Design review of the part built by this model. Coordinates are the model's own, in mm. Face numbers are marked on the shaded views. A direction names the side the tool comes from. Give positions to 0.01 mm unless a question says otherwise; leave off trailing zeros. Write each loop counter-clockwise with the first axis right and the second up, starting at its lowest first coordinate (ties: lowest second). Pieces come first, ordered by that corner, then holes. Notation, with made-up numbers: M -24.75,53.25 L -12.75,53.25 A7 cw -12.75,58.25 Z; hole C 73,78 d1. An arc over 180 degrees is marked long. One line per item, written item: value. Start each with the question number.
```python
from build123d import *

# Parameters (mm, degrees)
SKETCH1_W            = 300
SKETCH1_H            = 20
BOSS_EXTRUDE1_DEPTH  = 8
SKETCH2_W            = 34
SKETCH2_H            = 8
BOSS_EXTRUDE2_DEPTH  = 9
SKETCH3_W            = 34
SKETCH3_H            = 8
BOSS_EXTRUDE3_DEPTH  = 9
SKETCH4_R            = 1.45
CUT_EXTRUDE1_DEPTH   = 302.504560496
SKETCH5_W            = 25
SKETCH5_H            = 8
BOSS_EXTRUDE4_DEPTH  = 17
SKETCH6_W            = 25
SKETCH6_H            = 8
BOSS_EXTRUDE5_DEPTH  = 17
SKETCH7_W            = 10
SKETCH7_H            = 38
CUT_EXTRUDE2_DEPTH   = 303.37890138
SKETCH8_W            = 7
SKETCH8_H            = 16
CUT_EXTRUDE3_DEPTH   = 4
CUT_EXTRUDE4_DEPTH   = 7
BOSS_EXTRUDE6_DEPTH  = 10
SKETCH12_W           = 8
SKETCH12_H           = 8
BOSS_EXTRUDE7_DEPTH  = 17
SKETCH13_R           = 1.7
CUT_EXTRUDE6_DEPTH   = 305.926220585
SKETCH14_W           = 20
SKETCH14_H           = 12
BOSS_EXTRUDE8_DEPTH  = 10
SKETCH15_R           = 1.6
CUT_EXTRUDE7_DEPTH   = 20
SKETCH16_W           = 20
SKETCH16_H           = 12
BOSS_EXTRUDE9_DEPTH  = 10
SKETCH17_R           = 1.6
CUT_EXTRUDE8_DEPTH   = 20
SKETCH18_W           = 20
SKETCH18_H           = 12
BOSS_EXTRUDE10_DEPTH = 10
CUT_EXTRUDE9_START   = -20
SKETCH19_R           = 1.6
CUT_EXTRUDE9_DEPTH   = 20
SKETCH20_W           = 20
SKETCH20_H           = 12
BOSS_EXTRUDE11_DEPTH = 10
CUT_EXTRUDE10_START  = -20
SKETCH21_R           = 1.6
CUT_EXTRUDE10_DEPTH  = 20
SKETCH22_W           = 207
SKETCH22_H           = 50
BOSS_EXTRUDE12_DEPTH = 8
SKETCH23_W           = 191
SKETCH23_H           = 44
CUT_EXTRUDE11_DEPTH  = 4
SKETCH24_W           = 10
SKETCH24_H           = 44
BOSS_EXTRUDE14_DEPTH = 19.4
SKETCH25_R           = 1.45
CUT_EXTRUDE12_DEPTH  = 15
FILLET1_R            = 5
FILLET2_R            = 5
FILLET3_R            = 8
FILLET4_R            = 15
FILLET5_R            = 25
FILLET6_R            = 3
SKETCH27_W           = 1.8
SKETCH27_H           = 5
CUT_EXTRUDE13_DEPTH  = 19.4


with BuildPart() as part:
    # Sketch1 → Boss-Extrude1 (new body)
    with BuildSketch(Plane(origin=(0, 0, 0), x_dir=(1, 0, 0), z_dir=(0, 1, 0))):
        with Locations((150, -10)):
            Rectangle(SKETCH1_W, SKETCH1_H)
    extrude(amount=BOSS_EXTRUDE1_DEPTH)

    # Sketch2 → Boss-Extrude2 (add)
    with BuildSketch(Plane.XY.offset(20)):
        with Locations((17, 4)):
            Rectangle(SKETCH2_W, SKETCH2_H)
        with Locations((283, 4)):
            Rectangle(SKETCH2_W, SKETCH2_H)
    extrude(amount=BOSS_EXTRUDE2_DEPTH)

    # Sketch3 → Boss-Extrude3 (add)
    with BuildSketch(Plane(origin=(0, 0, 0), x_dir=(-1, 0, 0), z_dir=(0, 0, -1))):
        with Locations((-17, 4)):
            Rectangle(SKETCH3_W, SKETCH3_H)
        with Locations((-283, 4)):
            Rectangle(SKETCH3_W, SKETCH3_H)
    extrude(amount=BOSS_EXTRUDE3_DEPTH)

    # Sketch4 → Cut-Extrude1 (cut, through all)
    with BuildSketch(Plane(origin=(0, 8, 0), x_dir=(1, 0, 0), z_dir=(0, 1, 0))):
        with Locations(Location((4, 5, 0), (0, 0, 270))):
            Circle(SKETCH4_R)
        with Locations(Location((30, 5, 0), (0, 0, 270))):
            Circle(SKETCH4_R)
        with Locations(Location((30, -25, 0), (0, 0, 270))):
            Circle(SKETCH4_R)
        with Locations(Location((4, -25, 0), (0, 0, 270))):
            Circle(SKETCH4_R)
        with Locations(Location((296, -25, 0), (0, 0, 270))):
            Circle(SKETCH4_R)
        with Locations(Location((296, 5, 0), (0, 0, 270))):
            Circle(SKETCH4_R)
        with Locations(Location((270, -25, 0), (0, 0, 270))):
            Circle(SKETCH4_R)
        with Locations(Location((270, 5, 0), (0, 0, 270))):
            Circle(SKETCH4_R)
    extrude(amount=-CUT_EXTRUDE1_DEPTH, mode=Mode.SUBTRACT)

    # Sketch5 → Boss-Extrude4 (add)
    with BuildSketch(Plane.XY.offset(20)):
        with Locations((253.5, 4)):
            Rectangle(SKETCH5_W, SKETCH5_H)
    extrude(amount=BOSS_EXTRUDE4_DEPTH)

    # Sketch6 → Boss-Extrude5 (add)
    with BuildSketch(Plane(origin=(0, 0, 0), x_dir=(-1, 0, 0), z_dir=(0, 0, -1))):
        with Locations((-253.5, 4)):
            Rectangle(SKETCH6_W, SKETCH6_H)
    extrude(amount=BOSS_EXTRUDE5_DEPTH)

    # Sketch7 → Cut-Extrude2 (cut, through all)
    with BuildSketch(Plane(origin=(0, 8, 0), x_dir=(1, 0, 0), z_dir=(0, 1, 0))):
        with Locations((254, -10)):
            Rectangle(SKETCH7_W, SKETCH7_H)
    extrude(amount=-CUT_EXTRUDE2_DEPTH, mode=Mode.SUBTRACT)

    # Sketch8 → Cut-Extrude3 (cut)
    with BuildSketch(Plane(origin=(0, 8, 0), x_dir=(1, 0, 0), z_dir=(0, 1, 0))):
        with Locations((262.5, -10)):
            Rectangle(SKETCH8_W, SKETCH8_H)
    extrude(amount=-CUT_EXTRUDE3_DEPTH, mode=Mode.SUBTRACT)

    # Sketch9 → Cut-Extrude4 (cut)
    with BuildSketch(Plane.ZY.offset(-259)):
        Polygon((18, 4), (22, 8), (18, 8), align=None)
        Polygon((2, 4), (-2, 8), (2, 8), align=None)
    extrude(amount=-CUT_EXTRUDE4_DEPTH, mode=Mode.SUBTRACT)

    # Sketch10 → Boss-Extrude6 (add)
    with BuildSketch(Plane.ZY.offset(-259)):
        Polygon((-2, 0), (-9, 8), (-9, 0), align=None)
        Polygon((29, 8), (22, 0), (29, 0), align=None)
    extrude(amount=BOSS_EXTRUDE6_DEPTH)

    # Sketch12 → Boss-Extrude7 (add)
    with BuildSketch(Plane.XY.offset(37)):
        with Locations((245, 4)):
            Rectangle(SKETCH12_W, SKETCH12_H)
    extrude(amount=BOSS_EXTRUDE7_DEPTH)

    # Sketch13 → Cut-Extrude6 (cut, through all)
    with BuildSketch(Plane(origin=(0, 8, 0), x_dir=(1, 0, 0), z_dir=(0, 1, 0))):
        with Locations(Location((245, -50, 0), (0, 0, 270))):
            Circle(SKETCH13_R)
        with Locations(Location((245, -18, 0), (0, 0, 270))):
            Circle(SKETCH13_R)
    extrude(amount=-CUT_EXTRUDE6_DEPTH, mode=Mode.SUBTRACT)

    # Sketch14 → Boss-Extrude8 (add)
    with BuildSketch(Plane.XY.offset(29)):
        with Locations((285, 6)):
            Rectangle(SKETCH14_W, SKETCH14_H)
    extrude(amount=BOSS_EXTRUDE8_DEPTH)

    # Sketch15 → Cut-Extrude7 (cut)
    with BuildSketch(Plane(origin=(295, 0, 0), x_dir=(0, 0, -1), z_dir=(1, 0, 0))):
        with Locations((-35, 8)):
            Circle(SKETCH15_R)
    extrude(amount=-CUT_EXTRUDE7_DEPTH, mode=Mode.SUBTRACT)

    # Sketch16 → Boss-Extrude9 (add)
    with BuildSketch(Plane(origin=(0, 0, -9), x_dir=(-1, 0, 0), z_dir=(0, 0, -1))):
        with Locations((-285, 6)):
            Rectangle(SKETCH16_W, SKETCH16_H)
    extrude(amount=BOSS_EXTRUDE9_DEPTH)

    # Sketch17 → Cut-Extrude8 (cut)
    with BuildSketch(Plane(origin=(295, 0, 0), x_dir=(0, 0, -1), z_dir=(1, 0, 0))):
        with Locations((15, 8)):
            Circle(SKETCH17_R)
    extrude(amount=-CUT_EXTRUDE8_DEPTH, mode=Mode.SUBTRACT)

    # Sketch18 → Boss-Extrude10 (add)
    with BuildSketch(Plane(origin=(0, 0, -9), x_dir=(-1, 0, 0), z_dir=(0, 0, -1))):
        with Locations((-15, 6)):
            Rectangle(SKETCH18_W, SKETCH18_H)
    extrude(amount=BOSS_EXTRUDE10_DEPTH)

    # Sketch19 → Cut-Extrude9 (cut)
    with BuildSketch(Plane.ZY.offset(-5).offset(CUT_EXTRUDE9_START)):
        with Locations(Location((-15, 8, 0), (0, 0, 180))):
            Circle(SKETCH19_R)
    extrude(amount=CUT_EXTRUDE9_DEPTH, mode=Mode.SUBTRACT)

    # Sketch20 → Boss-Extrude11 (add)
    with BuildSketch(Plane.XY.offset(29)):
        with Locations((15, 6)):
            Rectangle(SKETCH20_W, SKETCH20_H)
    extrude(amount=BOSS_EXTRUDE11_DEPTH)

    # Sketch21 → Cut-Extrude10 (cut)
    with BuildSketch(Plane.ZY.offset(-5).offset(CUT_EXTRUDE10_START)):
        with Locations(Location((35, 8, 0), (0, 0, 180))):
            Circle(SKETCH21_R)
    extrude(amount=CUT_EXTRUDE10_DEPTH, mode=Mode.SUBTRACT)

    # Sketch22 → Boss-Extrude12 (add)
    with BuildSketch(Plane(origin=(0, 0, 0), x_dir=(-1, 0, 0), z_dir=(0, -1, 0))):
        with Locations((-137.5, -45)):
            Rectangle(SKETCH22_W, SKETCH22_H)
        with Locations((-137.5, 25)):
            Rectangle(SKETCH22_W, SKETCH22_H)
    extrude(amount=-BOSS_EXTRUDE12_DEPTH)

    # Sketch23 → Cut-Extrude11 (cut)
    with BuildSketch(Plane(origin=(0, 8, 0), x_dir=(1, 0, 0), z_dir=(0, 1, 0))):
        with Locations((137.5, -42)):
            Rectangle(SKETCH23_W, SKETCH23_H)
        with Locations((137.5, 22)):
            Rectangle(SKETCH23_W, SKETCH23_H)
    extrude(amount=-CUT_EXTRUDE11_DEPTH, mode=Mode.SUBTRACT)

    # Sketch24 → Boss-Extrude14 (add)
    with BuildSketch(Plane(origin=(0, 4, 0), x_dir=(1, 0, 0), z_dir=(0, 1, 0))):
        with Locations((103.4, -42)):
            Rectangle(SKETCH24_W, SKETCH24_H)
        with Locations((52, -42)):
            Rectangle(SKETCH24_W, SKETCH24_H)
    extrude(amount=BOSS_EXTRUDE14_DEPTH)

    # Sketch25 → Cut-Extrude12 (cut)
    with BuildSketch(Plane(origin=(0, 23.4, 0), x_dir=(1, 0, 0), z_dir=(0, 1, 0))):
        with Locations(Location((102.6, -49, 0), (0, 0, 270))):
            Circle(SKETCH25_R)
        with Locations(Location((102.6, -39, 0), (0, 0, 270))):
            Circle(SKETCH25_R)
        with Locations(Location((52.8, -49, 0), (0, 0, 270))):
            Circle(SKETCH25_R)
        with Locations(Location((52.8, -39, 0), (0, 0, 270))):
            Circle(SKETCH25_R)
    extrude(amount=-CUT_EXTRUDE12_DEPTH, mode=Mode.SUBTRACT)

    # Fillet1
    fillet1_edges = [part.edges().sort_by_distance(p)[0] for p in [
        (103.4, 8, 64),
        (103.4, 8, 20),
        (52, 8, 64),
        (52, 8, 20),
    ]]
    fillet(fillet1_edges, radius=FILLET1_R)

    # Fillet2
    fillet2_edges = [part.edges().sort_by_distance(p)[0] for p in [
        (47, 4, 42),
        (108.4, 4, 42),
    ]]
    fillet(fillet2_edges, radius=FILLET2_R - 0.0001)  # a hair under: the kernel refuses the full size

    # Fillet3
    fillet3_edges = [part.edges().sort_by_distance(p)[0] for p in [
        (241, 4, 54),
    ]]
    fillet(fillet3_edges, radius=FILLET3_R - 0.0001)  # a hair under: the kernel refuses the full size

    # Fillet4
    fillet4_edges = [part.edges().sort_by_distance(p)[0] for p in [
        (249, 4, 37),
    ]]
    fillet(fillet4_edges, radius=FILLET4_R)

    # Fillet5
    fillet5_edges = [part.edges().sort_by_distance(p)[0] for p in [
        (241, 4, -17),
    ]]
    fillet(fillet5_edges, radius=FILLET5_R - 0.0001)  # a hair under: the kernel refuses the full size

    # Fillet6
    fillet6_edges = [part.edges().sort_by_distance(p)[0] for p in [
        (285, 12, 29),
        (285, 12, 39),
        (285, 12, -9),
        (285, 12, -19),
        (15, 12, -9),
        (15, 12, -19),
        (15, 12, 29),
        (15, 12, 39),
    ]]
    fillet(fillet6_edges, radius=FILLET6_R)

    # Sketch27 → Cut-Extrude13 (cut)
    with BuildSketch(Plane(origin=(0, 23.4, 0), x_dir=(1, 0, 0), z_dir=(0, 1, 0))):
        with Locations((56.1, -44.5)):
            Rectangle(SKETCH27_W, SKETCH27_H)
        with Locations((99.3, -44.5)):
            Rectangle(SKETCH27_W, SKETCH27_H)
    extrude(amount=-CUT_EXTRUDE13_DEPTH, mode=Mode.SUBTRACT)


solid = part.part
```
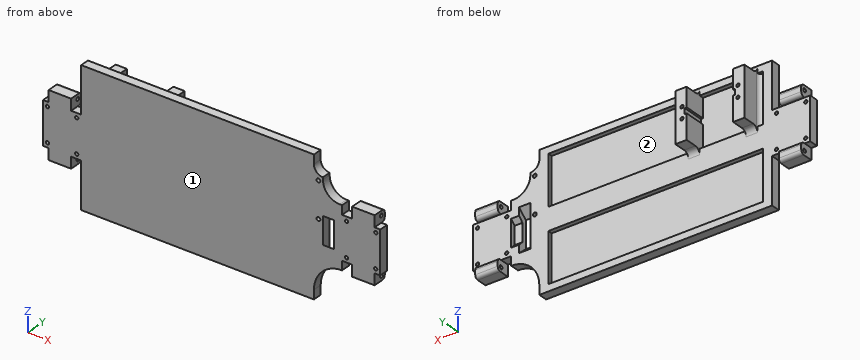
Q1. Machinability: for the marked faces 1 and 2, which of the approach directions +Z, -Z, +X, -X, +Y, -Y give a long, thin tool a straight path to every point of the face, cutting with its end or side? Answer none if there is none.
Q2. Wall thickness on line 1 (X direction, y = 2.75, z = 18); line 2 (X direction, y = 9.75, z = 31.5); line 3 (X direction, y = 15, z = 39): over which ranges is each line inside the solid? List them lowest first. Write a range as from..to.
Q3. Take a section at D-D, the plane z = -26. Give the boundary of the cut face in (x, y).
Q4. Take a section at A-A, the plane y = 17.25. Give the boundary of the cut face in (x, z).
Q5. For P1, Ø1.2, axis at y = 5.5, z = -22.5, coming from the -X side; P2, Ø0.9, axis at x = 56.5, y = 16, coming from the -Z side; P3, Ø10, axis at x = 233, y = 12, coming from the -Z side; P4, Ø9, axis at x = 269.5, y = 5, coming from the +Z side, all flat-tipped, find the tip position at first contact; note any pin that passes through.
Q6. Take a section at C-C, the plane x = 65. Give the boundary of the cut face in (y, z).
Q7. Take a section at B-B, the plane z = 6. Give the boundary of the cut face in (x, y).
Results list:
1. face 1: +Z, -Z, +X, -X, -Y
1. face 2: +Y
2. line 1: x = 0..243.3, 246.7..249, 259..300
2. line 2: x = 5..25, 47..57, 98.4..108.4, 275..295
2. line 3: x = 47..51.35, 54.25..57, 98.4..101.15, 104.05..108.4
3. outline: M 34,0 L 246.79,0 L 246.79,8 L 233,8 L 233,4 L 42,4 L 42,8 L 34,8 Z
4. outline: M 47,20 L 57,20 L 57,42 L 55.2,42 L 55.2,47 L 57,47 L 57,64 L 47,64 Z; M 98.4,20 L 108.4,20 L 108.4,64 L 98.4,64 L 98.4,47 L 100.2,47 L 100.2,42 L 98.4,42 Z; hole C 52.8,39 d2.9; hole C 52.8,49 d2.9; hole C 102.6,39 d2.9; hole C 102.6,49 d2.9
5. P1: stops at x = 34
5. P2: stops at z = 20
5. P3: stops at z = -50
5. P4: stops at z = 37
6. outline: M 0,-50 L 8,-50 L 8,-44 L 4,-44 L 4,0 L 8,0 L 8,20 L 4,20 L 4,64 L 8,64 L 8,70 L 0,70 Z
7. outline: M 0,0 L 249,0 L 249,8 L 0,8 Z; M 259,0 L 300,0 L 300,8 L 266,8 L 266,4 L 259,4 Z
